Part print with two shaded views. Sizes in mm from the minimum x, y, z corner. Coordinates: 2 decimals unless noted, no trailing zeros. Order: outer loops, then holes, each group sorted by start corner. A loop starts at its lowest first (then second) coordinate and runs counter-clockwise, first axis right, second up. Notation, with made-up numbers: (76, 35) - (119, 35) arc R34 cw to (119, 70) - close; hole circle Ø2 at (72, 4). An arc over 180 degrees is marked (long way). One line per item, written item: value.
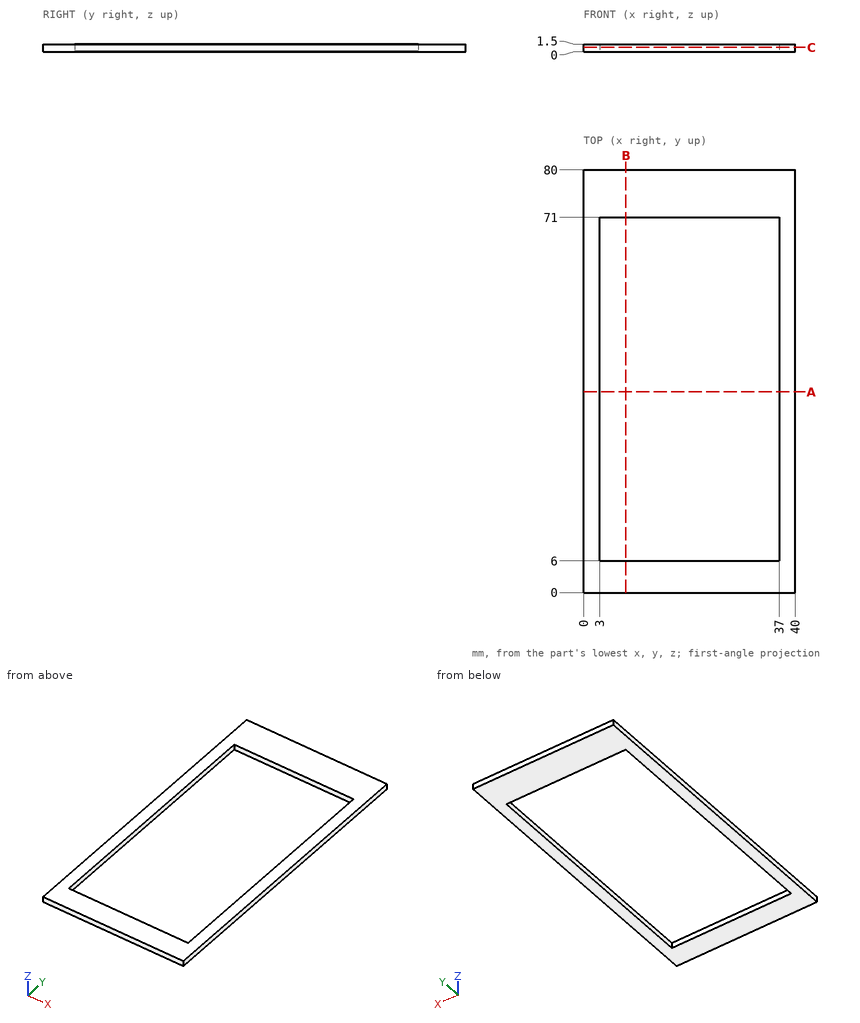
1. Band-saw the part on B-B, the plane x = 8. Give the cut face in (y, z), and give its area (3 significant figures).
Values found:
outline: (0, 0) - (6, 0) - (6, 1.5) - (0, 1.5) - close; (71, 0) - (80, 0) - (80, 1.5) - (71, 1.5) - close
area: 22.5 mm2
2. Probe line 1 along Y through (x, z) = (6.5, 0.75); line 2 along X through (y, z) = (15, 1.1). List the from-to ranges inside material, lowest first.
Values found:
line 1: y = 0 to 6, 71 to 80
line 2: x = 0 to 3, 37 to 40
3. Band-saw the part on A-A, the plane y = 38. Give the cut face in (x, z), and give its area (3 significant figures).
Values found:
outline: (0, 0) - (3, 0) - (3, 1.5) - (0, 1.5) - close; (37, 0) - (40, 0) - (40, 1.5) - (37, 1.5) - close
area: 9.00 mm2
4. Band-saw the part on C-C, the plane z = 0.85. Give the cut face in (x, y), and give its area (3 significant figures).
Values found:
outline: (0, 0) - (40, 0) - (40, 80) - (0, 80) - close; hole (3, 6) - (37, 6) - (37, 71) - (3, 71) - close
area: 990 mm2
